```python
from build123d import *

# Parameters (mm, degrees)
SZKIC1_W                    = 15
SZKIC1_H                    = 7
SZKIC1_R                    = 1.5
DODANIE_WYCI_GNI_CIE2_DEPTH = 3
SZKIC2_R                    = 1.5
DODANIE_WYCI_GNI_CIE3_DEPTH = 15


with BuildPart() as part:
    # Szkic1 → Dodanie-wyciągnięcie2 (new body)
    with BuildSketch(Plane.XY):
        Rectangle(SZKIC1_W, SZKIC1_H)
        with Locations((-3.25, 0)):
            Circle(SZKIC1_R, mode=Mode.SUBTRACT)
        with Locations((3.25, 0)):
            Circle(SZKIC1_R, mode=Mode.SUBTRACT)
    extrude(amount=DODANIE_WYCI_GNI_CIE2_DEPTH)

    # Szkic2 → Dodanie-wyciągnięcie3 (add)
    with BuildSketch(Plane(origin=(7.5, 0, 0), x_dir=(0, 0, -1), z_dir=(1, 0, 0))):
        with BuildLine():
            Line((0, -3.5), (0.074433096, -6.499076619))
            ThreePointArc((0.074433096, -6.499076619), (-5.147475229, -8.776813713), (-3, -3.5))
            Line((-3, -3.5), (0, -3.5))
        make_face()
        with Locations((-3, -6.5)):
            Circle(SZKIC2_R, mode=Mode.SUBTRACT)
    extrude(amount=-DODANIE_WYCI_GNI_CIE3_DEPTH)


solid = part.part
```
Verification items for the finished model (mm, model axes). A direction names the side the tool comes from. Give positions to 0.01 mm unless a question says otherwise; leave off trailing zeros. Order: outer loops, then holes, each group sorted by start corner. A loop starts at its lowest first (then second) coordinate and runs counter-clockwise, first axis right, second up. Notation, with made-up numbers: M 4,-8.75 L 31,-8.75 A33 cw 31,25.25 Z; hole C 73,29 d3. An arc over 180 degrees is marked long. Return JSON: item names as keys, results as strings. Group by question number.
1) Section check B-B on x = 3.25. Record the cut outline in (y, z), and give its area (3 significant figures).
2) Scan lines: line 1 (X direction, y = -1, z = 0.5); line 2 (X direction, y = -1.25, z = 1.5); line 3 (Z direction, x = 2.5, y = -7.5). Record each from-to range of solid material in increasing order.
3) Mould release check, pull along Y, two halves, no side actions. Record for faces 1 (the face through (0.105, -7.075, 1.614)), 2 (the face through (0, 0, 3)), 3 (the face through (0, 3.5, 1)): pulls with the +Y half, pulls with the -Y half, needs draft (parallel to the pull), parting line crosses it, or undercut.
4) Section check C-C on y = -6.25. Record the cut outline in (x, z).
5) Section check A-A on z = 2. Record the cut outline in (x, y), and give its area (3 significant figures).
6) Access from +Z, -Z, +X, -X, +Y, -Y to the whole of each face (thin tool, end or side, straight path). Record for faces 4 (the face through (0, 0, 0)), 5 (the face through (-7.5, -3, 2)).
7) Section check D-D on x = -1.25. Record the cut outline in (y, z).
8) Go/stop test with flat-tipped pins: pin 1 Ø4 at (x, y) = (-3.25, 0) entering from +Z; pin 2 Ø3 at (x, y) = (-2, -3) entering from -Z; pin 3 Ø1 at (x, y) = (3, -5.5) entering from -Z. Record where each tip stops, or that it passes through.
Answer block:
{
 "1": {"outline": "M -6.5,-0.07 L -3.5,0 L -1.5,0 L -1.5,3 L -3.5,3 A3.08 ccw long Z; M 1.5,0 L 3.5,0 L 3.5,3 L 1.5,3 Z; hole C -6.5,3 d3", "area": "36.6 mm^2"},
 "2": {"line 1": "x = -7.5 to -4.37, -2.13 to 2.13, 4.37 to 7.5", "line 2": "x = -7.5 to -4.08, -2.42 to 2.42, 4.08 to 7.5", "line 3": "z = 0.07 to 1.88, 4.12 to 5.93"},
 "3": {"face 1": "undercut", "face 2": "needs draft", "face 3": "pulls with the +Y half"},
 "4": {"outline": "M -7.5,-0.07 L 7.5,-0.07 L 7.5,1.52 L -7.5,1.52 Z; M -7.5,4.48 L 7.5,4.48 L 7.5,6.06 L -7.5,6.06 Z"},
 "5": {"outline": "M -7.5,-9.48 L 7.5,-9.48 L 7.5,-7.62 L -7.5,-7.62 Z; M -7.5,-5.38 L 7.5,-5.38 L 7.5,3.5 L -7.5,3.5 Z; hole C -3.25,0 d3; hole C 3.25,0 d3", "area": "147 mm^2"},
 "6": {"face 4": "-Z, +X, -X, +Y", "face 5": "+Z, -Z, -X, +Y, -Y"},
 "7": {"outline": "M -6.5,-0.07 L -3.5,0 L 3.5,0 L 3.5,3 L -3.5,3 A3.08 ccw long Z; hole C -6.5,3 d3"},
 "8": {"pin 1": "stops at z = 3", "pin 2": "stops at z = -0.02", "pin 3": "stops at z = -0.06"}
}
